Work out the finished part from the listing and answer in its coordinate system (mm). A direction names the side the tool comes from. Coordinates: 2 decimals unless noted, no trailing zeros. Order: outer loops, then holes, each group sorted by start corner. A loop starts at its lowest first (then second) coordinate and runs counter-clockwise, first axis right, second up. Notation, with made-up numbers: (-32.75, 0) -> (12.25, 0) arc R20 ccw to (12.25, 19) -> close; hole circle Ø9 at (78, 88). An arc over 180 degrees is marked (long way). Write item = value, one per line. Start each with the question number.
Q1. The part is cut by section B-B, the plane y = -23. Determine the outline of the cut face in (x, z).
Q2. Straight lines are drawn through the part: L1, parallel to X at y = -19, z = 37.5; L2, parallel to X at y = -30.5, z = 22; L3, parallel to Y at x = 42, z = 31. For each, find the intervals that lie inside material, in ascending order. Write a range as from..to.
Q3. The part is cut by section C-C, the plane x = 39.5. Determine the outline of the cut face in (y, z), plus the area to 3 significant figures.
Q4. The part is cut by section D-D, the plane z = 8. Determine the outline of the cut face in (x, y).
Q5. The part is cut by section A-A, the plane z = 23.5. Determine the outline of the cut face in (x, y).
Q6. Which of the six approach directions +Z, -Z, +X, -X, +Y, -Y give full straight-line access (tool end or side, diameter ignored) to faces 1 (the flat face through (8, -25, 45)), 2 (the flat face through (20, -30, 45)), 3 (the flat face through (39, -10, 35)), 4 (the flat face through (47, -40, 40))?
Q7. For a pull along Y with two mould halves and no side action, classify faces 5 (the cylindrical face through (17.482, -32.129, 12.325)), 6 (the flat face through (25, -14, 50)), 7 (the cylindrical face through (10.49, -39.28, 45.07)) as +Y half, -Y half, draft (parallel to the pull), parting line (faces both ways), or undercut.
Q8. Flat-ended cylindrical pins translate along their axes: pin 1 (2 mm diameter, centred on x = 17.5, z = 44.5, fed in from -Y); pin 2 (3 mm diameter, centred on x = 39, y = -29.5, fed in from +Z); pin 3 (3 mm diameter, centred on x = 37.5, z = 42, fed in from -Y). Find the tip coordinate at first contact, or state that the pin passes through.
```python
from build123d import *

# Parameters (mm, degrees)
F0_W      = 50
F0_H      = 50
F1_DEPTH  = 50
F3_DEPTH  = 6
F5_DEPTH  = 40
F6_R      = 10
F8_DEPTH  = 10
F10_DEPTH = 25


with BuildPart() as f1:
    # F0 (on Front) → F1 (new body)
    with BuildSketch(Plane.XZ):
        with Locations((25, 25)):
            Rectangle(F0_W, F0_H)
    extrude(amount=F1_DEPTH)

    # F2 (on face) → F3 (cut)
    with BuildSketch(Plane.YZ.offset(50)):
        Polygon((-30, 50), (-50, 50), (-50, 30), align=None)
    extrude(amount=-F3_DEPTH, mode=Mode.SUBTRACT)

    # F4 (on face) → F5 (cut)
    with BuildSketch(Plane.XZ.offset(50)):
        Polygon((44, 30), (44, 50), (34, 50), (34, 10), (44, 10), align=None)
    extrude(amount=-F5_DEPTH, mode=Mode.SUBTRACT)

    # F6
    f6_edges = [f1.edges().sort_by_distance(p)[0] for p in [
        (39, -10, 10),
    ]]
    fillet(f6_edges, radius=F6_R)

    # F7 (on face) → F8 (cut)
    with BuildSketch(Plane.XY.offset(50)):
        with BuildLine():
            ThreePointArc((0, -35), (10.6066017178, -39.3933982822), (15, -50))
            Line((15, -50), (25, -50))
            Line((25, -50), (25, -35))
            Line((25, -35), (15, -25))
            Line((15, -25), (0, -25))
            Line((0, -25), (0, -35))
        make_face()
    extrude(amount=-F8_DEPTH, mode=Mode.SUBTRACT)

    # F9 (on face) → F10 (cut)
    with BuildSketch(Plane(origin=(0, 0, 0), x_dir=(1, 0, 0), z_dir=(0, 0, -1))):
        with BuildLine():
            ThreePointArc((0, 25), (17.6776695297, 32.3223304703), (25, 50))
            Line((25, 50), (0, 50))
            Line((0, 50), (0, 25))
        make_face()
    extrude(amount=-F10_DEPTH, mode=Mode.SUBTRACT)

    # F12 (on face) + F13 (on face) → F14 (revolve, cut)
    with BuildSketch(Plane.XZ.offset(50)):
        Polygon((25, 25), (0, 50), (0, 25), align=None)
    with BuildSketch(Plane(origin=(0, 0, 0), x_dir=(0, -1, 0), z_dir=(-1, 0, 0))):
        Polygon((50, 25), (50, 50), (25, 25), align=None)
    revolve(axis=Axis((0, -50, 25), (0, 0, -1)), mode=Mode.SUBTRACT)


solid = f1.part
```
Model answer:
q1.outline = (0, 0) -> (50, 0) -> (50, 50) -> (44, 50) -> (44, 10) -> (34, 10) -> (34, 50) -> (0, 50) -> close
q2.L1 = 0..34, 44..50
q2.L2 = 15.64..34, 44..50
q2.L3 = -10..0
q3.outline = (-50, 0) -> (0, 0) -> (0, 50) -> (-10, 50) -> (-10, 20) arc R10 cw to (-20, 10) -> (-50, 10) -> close
q3.area = 921 mm2
q4.outline = (0, -25) arc R25 cw to (25, -50) -> (50, -50) -> (50, 0) -> (0, 0) -> close
q5.outline = (0, -25) arc R25 cw to (25, -50) -> (34, -50) -> (34, -10) -> (44, -10) -> (44, -50) -> (50, -50) -> (50, 0) -> (0, 0) -> close
q6.face_1 = +Z, -X
q6.face_2 = +Z, -X, -Y
q6.face_3 = +Z, -Y
q6.face_4 = +Z, +X, -Y
q7.face_5 = -Y half
q7.face_6 = draft
q7.face_7 = undercut
q8.pin_1 = -28.5
q8.pin_2 = 10
q8.pin_3 = -10
